For this review, take the finished solid that the model builds, in its own axes (mm). Face numbers are marked on the shaded views. A direction names the side the tool comes from. Give positions to 0.01 mm unless a question says otherwise; leave off trailing zeros. Write each loop counter-clockwise with the first axis right and the second up, starting at its lowest first coordinate (ties: lowest second). Pieces come first, ordered by that corner, then holes.
Q1. We need section D-D (z = -4.5). Give the number of separate pieces and of enclosed holes in the cut face, then the cut area to 3 significant figures.
Q2. We need section A-A (y = 4). Write out the cut boundary in (x, z) (3 decimals).
Q3. Insertion check: P1, Ø3.5, axis at x = 0, z = 9, coming from the -Y side; P2, Ø2, axis at y = 2.5, z = -2.5, coming from the +X side; P3, Ø1, axis at x = -10, y = 6, coming from the -Z side; P4, Ø3, axis at y = 3.5, z = -2.5, coming from the +X side. Each pin has a flat end and moves straight along its axis. Give the tip position at first contact, or say it passes through.
Q4. We need section C-C (y = 6.25). Write out the cut boundary in (x, z) (3 decimals), then the cut area to 3 significant figures.
Q5. Mouldability with a two-part tool opening along X and no side actions: class the marked faces 4, 5 and 6 as released by +X, released by -X, zero draft, split by the parting line, or undercut.
Q6. Machinability: for the marked faces 1, 2 and 3, which of the approach directions +Z, -Z, +X, -X, +Y, -Y give a long, thin tool a straight path to every point of the face, cutting with its end or side? Answer none if there is none.
Q7. We need section B-B (z = 0). Write out the cut boundary in (x, y) (3 decimals), then the cut area to 3 significant figures.
Q8. For line 1 (Z direction, x = 1, y = 0.5); line 2 (Z direction, x = 8.75, y = 3.25); line 3 (Z direction, x = 9, y = 4.75), list the stretches that pass through material, from the lowest coordinate up.
```python
from build123d import *

# Parameters (mm, degrees)
SKETCH1_R                      = 14.5
BOSS_EXTRUDE1_DEPTH            = 9.525
SKETCH2_R                      = 3.5
CUT_EXTRUDE1_DEPTH             = 3.5
SKETCH3_R                      = 3.125
CUT_EXTRUDE2_DEPTH             = 5
CBORE_FOR_M4_SHCS1_D           = 4.3
CBORE_FOR_M4_SHCS1_CBORE_D     = 8
CBORE_FOR_M4_SHCS1_CBORE_DEPTH = 4
CIRPATTERN1_COUNT              = 3
FILLET1_R                      = 5
CUT_EXTRUDE3_DEPTH             = 5
CIRPATTERN2_COUNT              = 3


with BuildPart() as part:
    # Sketch1 → Boss-Extrude1 (new body)
    with BuildSketch(Plane(origin=(0, 0, 0), x_dir=(1, 0, 0), z_dir=(0, 1, 0))):
        with Locations(Location((0, 0, 0), (0, 0, 90))):
            Circle(SKETCH1_R)
    extrude(amount=BOSS_EXTRUDE1_DEPTH)

    # Sketch2 → Cut-Extrude1 (cut)
    with BuildSketch(Plane.XZ):
        with Locations(Location((0, 0, 0), (0, 0, 270))):
            Circle(SKETCH2_R)
    extrude(amount=-CUT_EXTRUDE1_DEPTH, mode=Mode.SUBTRACT)

    # Sketch3 → Cut-Extrude2 (cut)
    with BuildSketch(Plane.XZ.offset(-3.5)):
        with Locations(Location((0, 0, 0), (0, 0, 270))):
            Circle(SKETCH3_R)
    extrude(amount=-CUT_EXTRUDE2_DEPTH, mode=Mode.SUBTRACT)

    # CBORE for M4 SHCS1 (through all)
    with Locations(Plane(origin=(0, 9.525, 0), x_dir=(-1, 0, 0), z_dir=(0, 1, 0))):
        with Locations((0, 9)):
            cbore_for_m4_shcs1 = CounterBoreHole(CBORE_FOR_M4_SHCS1_D / 2, CBORE_FOR_M4_SHCS1_CBORE_D / 2, CBORE_FOR_M4_SHCS1_CBORE_DEPTH)

    # CirPattern1: CBORE for M4 SHCS1 ×3 about axis
    cirpattern1_axis = Axis((0, 0, 0), (0, 1, 0))
    for i in range(1, CIRPATTERN1_COUNT):
        add(cbore_for_m4_shcs1.rotate(cirpattern1_axis, i * 360 / CIRPATTERN1_COUNT), mode=Mode.SUBTRACT)

    # Fillet1
    # the kernel refuses this fillet: 5 mm, written as the material it takes off along each edge
    with BuildSketch(Plane(origin=(0, 9.525, 0), x_dir=(0, 0, -1), z_dir=(1, 0, 0))) as fillet1_piece_1:
        with BuildLine():
            CenterArc((14.5 - FILLET1_R, -FILLET1_R), FILLET1_R, 0, 90)
            Line((14.5 - FILLET1_R, 0), (14.5, 0))
            Line((14.5, 0), (14.5, -FILLET1_R))
        make_face()
    revolve(axis=Axis((0, 9.525, 0), (0, 1, 0)), mode=Mode.SUBTRACT)

    # Sketch6 → Cut-Extrude3 (cut)
    with BuildSketch(Plane.XZ):
        with BuildLine():
            ThreePointArc((-11.401615906, 1.501051211), (-9.249319233, -1.303876423), (-6.444391599, 0.848420249))
            ThreePointArc((-6.444391599, 0.848420249), (-5.629165125, 3.25), (-3.956949289, 5.156796712))
            ThreePointArc((-3.956949289, 5.156796712), (-3.49546951, 8.662083635), (-7.000756434, 9.123563413))
            ThreePointArc((-7.000756434, 9.123563413), (-9.959292144, 5.75), (-11.401615906, 1.501051211))
        make_face()
    cut_extrude3 = extrude(amount=-CUT_EXTRUDE3_DEPTH, mode=Mode.SUBTRACT)

    # CirPattern2: Cut-Extrude3 ×3 about axis
    cirpattern2_axis = Axis((0, 0, 0), (0, 1, 0))
    for i in range(1, CIRPATTERN2_COUNT):
        add(cut_extrude3.rotate(cirpattern2_axis, i * 360 / CIRPATTERN2_COUNT), mode=Mode.SUBTRACT)


solid = part.part
```
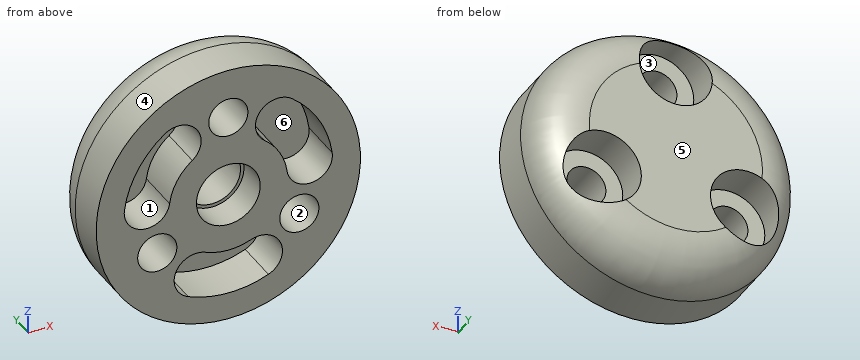
Computed:
1. separate pieces: 3
1. enclosed holes: 0
1. area: 142 mm2
2. outline: circle Ø29 at (0, 0); hole (-11.402, 1.501) arc R2.5 ccw to (-6.444, 0.848) arc R6.5 cw to (-3.957, 5.157) arc R2.5 ccw to (-7.001, 9.124) arc R11.5 ccw to start; hole circle Ø4.3 at (-7.794, -4.5); hole (-4.401, -10.625) arc R11.5 ccw to (4.401, -10.625) arc R2.5 ccw to (2.487, -6.005) arc R6.5 cw to (-2.487, -6.005) arc R2.5 ccw to start; hole circle Ø6.25 at (0, 0); hole circle Ø4.3 at (0, 9); hole (3.957, 5.157) arc R6.5 cw to (6.444, 0.848) arc R2.5 ccw to (11.402, 1.501) arc R11.5 ccw to (7.001, 9.124) arc R2.5 ccw to start; hole circle Ø4.3 at (7.794, -4.5)
3. P1: passes through
3. P2: stops at x = 14.42
3. P3: stops at z = -10.7
3. P4: stops at x = 14.47
4. outline: circle Ø28.386 at (0, 0); hole circle Ø8 at (-7.794, -4.5); hole circle Ø8 at (0, 9); hole circle Ø6.25 at (0, 0); hole circle Ø8 at (7.794, -4.5)
4. area: 451 mm2
5. face 4: split by the parting line
5. face 5: zero draft
5. face 6: undercut
6. face 1: -Y
6. face 2: +Y, -Y
6. face 3: +Y
7. outline: (-14.5, 0) - (-11.13, 0) - (-11.13, 5) - (-6.716, 5) - (-6.716, 0) - (-3.5, 0) - (-3.5, 3.5) - (-3.125, 3.5) - (-3.125, 8.5) - (3.125, 8.5) - (3.125, 3.5) - (3.5, 3.5) - (3.5, 0) - (6.716, 0) - (6.716, 5) - (11.13, 5) - (11.13, 0) - (14.5, 0) - (14.5, 4.525) arc R5 ccw to (9.5, 9.525) - (-9.5, 9.525) arc R5 ccw to (-14.5, 4.525) - close
7. area: 166 mm2
8. line 1: z = -14.47 to -11.46, -6.42 to -3.35, 3.35 to 7.1, 10.9 to 14.47
8. line 2: z = -11.56 to -6.43, -2.57 to -1.32, 7.46 to 11.56
8. line 3: z = -11.36 to -6.28, -2.72 to -1.32, 7.16 to 11.36
